```python
from build123d import *

# Parameters (mm, degrees)
SKETCH1_W                                           = 69.85
SKETCH1_H                                           = 44.45
BOSS_EXTRUDE1_DEPTH                                 = 39.6875
CBORE_FOR_10_BINDING_HEAD_MACHINE_SCREW_D           = 5.1054
CBORE_FOR_10_BINDING_HEAD_MACHINE_SCREW_CBORE_D     = 9.525
CBORE_FOR_10_BINDING_HEAD_MACHINE_SCREW_CBORE_DEPTH = 7.9375
FILLET2_R                                           = 6.35
F_1_4_0_25_DIAMETER_HOLE1_D                         = 6.35
SKETCH9_W                                           = 15.875
SKETCH9_H                                           = 15.875
CUT_EXTRUDE1_DEPTH                                  = 6.35
FILLET3_R                                           = 6.35
FILLET3_OF_MIRROR2_R                                = 6.35
MIRROR3_START                                       = 33.3375
MIRROR3_OUTLINE_R                                   = 3.175
MIRROR3_DEPTH                                       = 6.35


# Read off the part's stored shape, not the designer's step: Mirror3
with BuildPart() as part:
    # Sketch1 → Boss-Extrude1 (new body)
    with BuildSketch(Plane(origin=(0, 0, 0), x_dir=(1, 0, 0), z_dir=(0, 1, 0))):
        Rectangle(SKETCH1_W, SKETCH1_H)
    extrude(amount=BOSS_EXTRUDE1_DEPTH)

    # CBORE for #10 Binding Head Machine Screw1 (through all)
    with Locations(Plane(origin=(0, 0, 0), x_dir=(-1, 0, 0), z_dir=(0, -1, 0))):
        with Locations((-11.136931804, 11.136931804), (11.136931804, 11.136931804), (11.136931804, -11.136931804), (-11.136931804, -11.136931804)):
            CounterBoreHole(CBORE_FOR_10_BINDING_HEAD_MACHINE_SCREW_D / 2, CBORE_FOR_10_BINDING_HEAD_MACHINE_SCREW_CBORE_D / 2, CBORE_FOR_10_BINDING_HEAD_MACHINE_SCREW_CBORE_DEPTH)

    # Fillet2
    fillet2_edges = [part.edges().sort_by_distance(p)[0] for p in [
        (34.925, 19.84375, 22.225),
        (-34.925, 19.84375, 22.225),
        (-34.925, 19.84375, -22.225),
        (34.925, 19.84375, -22.225),
    ]]
    fillet(fillet2_edges, radius=FILLET2_R)

    # 1/4 (0.25) Diameter Hole1 (through all)
    with Locations(Plane(origin=(0, 39.6875, 0), x_dir=(-1, 0, 0), z_dir=(0, 1, 0))):
        with Locations((-28.575, -15.875), (-28.575, 15.875), (28.575, 15.875), (28.575, -15.875)):
            f_1_4_0_25_diameter_hole1 = Hole(F_1_4_0_25_DIAMETER_HOLE1_D / 2)

    # Mirror1: 1/4 (0.25) Diameter Hole1 across plane
    add(f_1_4_0_25_diameter_hole1.mirror(Plane(origin=(0, 0, 0), x_dir=(0, 0, 1), z_dir=(1, 0, 0))), mode=Mode.SUBTRACT)

    # Sketch9 → Cut-Extrude1 (cut)
    with BuildSketch(Plane(origin=(0, 39.6875, 0), x_dir=(1, 0, 0), z_dir=(0, 1, 0))):
        with Locations((-26.9875, 14.2875)):
            Rectangle(SKETCH9_W, SKETCH9_H)
    cut_extrude1 = extrude(amount=-CUT_EXTRUDE1_DEPTH, mode=Mode.SUBTRACT)

    # Fillet3
    fillet3_edges = [part.edges().sort_by_distance(p)[0] for p in [
        (-19.05, 36.5125, -6.35),
    ]]
    fillet(fillet3_edges, radius=FILLET3_R)

    # Mirror2: Cut-Extrude1 across plane
    add(cut_extrude1.mirror(Plane.XY), mode=Mode.SUBTRACT)

    # Fillet3 of Mirror2
    fillet3_of_mirror2_edges = [part.edges().sort_by_distance(p)[0] for p in [
        (-19.05, 36.5125, 6.35),
    ]]
    fillet(fillet3_of_mirror2_edges, radius=FILLET3_OF_MIRROR2_R)

    # Mirror3 outline → Mirror3 (cut)
    # profile 1 of 2: a face of its own
    with BuildSketch(Plane(origin=(0, 0, 0), x_dir=(1, 0, 0), z_dir=(0, 1, 0)).offset(MIRROR3_START)):
        with BuildLine():
            Line((25.4, 6.35), (34.925, 6.35))
            Line((34.925, 6.35), (34.925, 15.875))
            ThreePointArc((34.925, 15.875), (33.065128061, 20.365128061), (28.575, 22.225))
            Line((28.575, 22.225), (19.05, 22.225))
            Line((19.05, 22.225), (19.05, 12.7))
            ThreePointArc((19.05, 12.7), (20.909871939, 8.209871939), (25.4, 6.35))
        make_face()
        with Locations((28.575, 15.875)):
            Circle(MIRROR3_OUTLINE_R, mode=Mode.SUBTRACT)
    # profile 2 of 2: a face of its own
    with BuildSketch(Plane(origin=(0, 0, 0), x_dir=(1, 0, 0), z_dir=(0, 1, 0)).offset(MIRROR3_START)):
        with BuildLine():
            Line((34.925, -15.875), (34.925, -6.35))
            Line((34.925, -6.35), (25.4, -6.35))
            ThreePointArc((25.4, -6.35), (20.909871939, -8.209871939), (19.05, -12.7))
            Line((19.05, -12.7), (19.05, -22.225))
            Line((19.05, -22.225), (28.575, -22.225))
            ThreePointArc((28.575, -22.225), (33.065128061, -20.365128061), (34.925, -15.875))
        make_face()
        with Locations((28.575, -15.875)):
            Circle(MIRROR3_OUTLINE_R, mode=Mode.SUBTRACT)
    extrude(amount=MIRROR3_DEPTH, mode=Mode.SUBTRACT)


solid = part.part
```
Geometry check sheet. Reference: the model listing, model coordinates, mm. A direction names the side the tool comes from. Round coordinates to 2 decimals unless told otherwise and drop trailing zeros. Order: outer loops, then holes, each group sorted by start corner. A loop starts at its lowest first (then second) coordinate and runs counter-clockwise, first axis right, second up. Notation, with made-up numbers: (63, 49.25) - (99, 49.25) arc R12 ccw to (99, 61.25) - close; hole circle Ø2 at (-37.75, -25.75). An arc over 180 degrees is marked (long way). Use a Markdown table: item, result. Add a question column.
(1) Depth check by flat-ended pin: pin 1 (5 mm diameter, centred on x = -28, y = 37, fed in from -Z); pin 2 (5 mm diameter, centred on x = -27.5, z = -16, fed in from +Y); pin 3 (3 mm diameter, centred on x = -30, y = 37.5, fed in from +Z). Enter the tip coordinate at first touch or a pass-through.
(2) Release check for a two-part mould opening along X. For faces 4 (the flat face through (0, 39.688, 0)), 5 (the flat face through (9, 7.938, 13)), 6 (the flat face through (34.925, 20, 0)) record: pulls with the +X half, pulls with the -X half, needs draft (parallel to the pull), parting line crosses it, or undercut.
(3) Tool access check on faces 1 (the flat face through (25, 33.338, -14)), 2 (the cylindrical face through (20.96, 36.47, 8.16)), 3 (the cylindrical face through (-10.105, 3.913, 15.786)). Record the directions out of +Z, -Z, +X, -X, +Y, -Y that give a thin tool (end or side, any length) a straight path to the whole face; none if there is none.
(4) Sectioned sample at D-D, the plane y = 3.5. Count the separate pieces of the cut face and the enclosed holes in it, and give its area (3 significant figures).
(5) Sectioned sample at C-C, the plane x = -10. Enter the section's corners in (y, z) (1 decimal).
(6) Sectioned sample at A-A, the plane z = 17. Enter the section's corners in (x, y), and give its area (3 significant figures).
(7) Sectioned sample at B-B, the plane y = 37.5. Enter the section's corners in (x, z) (3 decimals).
(8) Material ranges on line 1 along Z through (x, y) = (11, 37.5) (3 decimals); line 2 along X through (y, z) = (8.5, 13) (3 decimals); line 3 along X through (y, z) = (29, -10) (3 decimals), recorded low to high. Write a range as [from, to].
Answers below:
| question | item | result |
|---|---|---|
| 1 | pin 1 | z = -6.35 |
| 1 | pin 2 | y = 33.34 |
| 1 | pin 3 | z = 6.35 |
| 2 | face 4 | needs draft |
| 2 | face 5 | undercut |
| 2 | face 6 | pulls with the +X half |
| 3 | face 1 | -Z, +X, +Y |
| 3 | face 2 | +Z, +X, +Y |
| 3 | face 3 | -Y |
| 4 | separate pieces | 1 |
| 4 | enclosed holes | 8 |
| 4 | area | 2,660 mm² |
| 5 | outline | (0, -22.2) - (39.7, -22.2) - (39.7, -13.4) - (7.9, -13.4) - (7.9, -15.8) - (0, -15.8) - close; (0, -6.5) - (7.9, -6.5) - (7.9, -8.9) - (39.7, -8.9) - (39.7, 8.9) - (7.9, 8.9) - (7.9, 6.5) - (0, 6.5) - close; (0, 15.8) - (7.9, 15.8) - (7.9, 13.4) - (39.7, 13.4) - (39.7, 22.2) - (0, 22.2) - close |
| 6 | outline | (-34.82, 0) - (-31.54, 0) - (-31.54, 33.34) - (-34.82, 33.34) - close; (-25.61, 0) - (25.61, 0) - (25.61, 33.34) - (19.05, 33.34) - (19.05, 39.69) - (-19.05, 39.69) - (-19.05, 33.34) - (-25.61, 33.34) - close; (31.54, 0) - (34.82, 0) - (34.82, 33.34) - (31.54, 33.34) - close |
| 6 | area | 2,170 mm² |
| 7 | outline | (-34.925, -6.35) - (-25.4, -6.35) arc R6.35 cw to (-19.05, -12.7) - (-19.05, -22.225) - (19.05, -22.225) - (19.05, -12.7) arc R6.35 cw to (25.4, -6.35) - (34.925, -6.35) - (34.925, 6.35) - (25.4, 6.35) arc R6.35 cw to (19.05, 12.7) - (19.05, 22.225) - (-19.05, 22.225) - (-19.05, 12.7) arc R6.35 cw to (-25.4, 6.35) - (-34.925, 6.35) - close; hole circle Ø5.105 at (-11.137, -11.137); hole circle Ø5.105 at (-11.137, 11.137); hole circle Ø5.105 at (11.137, -11.137); hole circle Ø5.105 at (11.137, 11.137) |
| 8 | line 1 | [-22.225, -13.686], [-8.588, 8.588], [13.686, 22.225] |
| 8 | line 2 | [-34.925, -29.922], [-27.228, -12.882], [-9.392, 9.392], [12.882, 27.228], [29.922, 34.925] |
| 8 | line 3 | [-34.925, -13.422], [-8.851, 8.851], [13.422, 34.925] |
